Verification items for this drawing (mm, ordinates from the low corner). A direction names the side the tool comes from. Coordinates: 2 decimals unless noted, no trailing zeros.
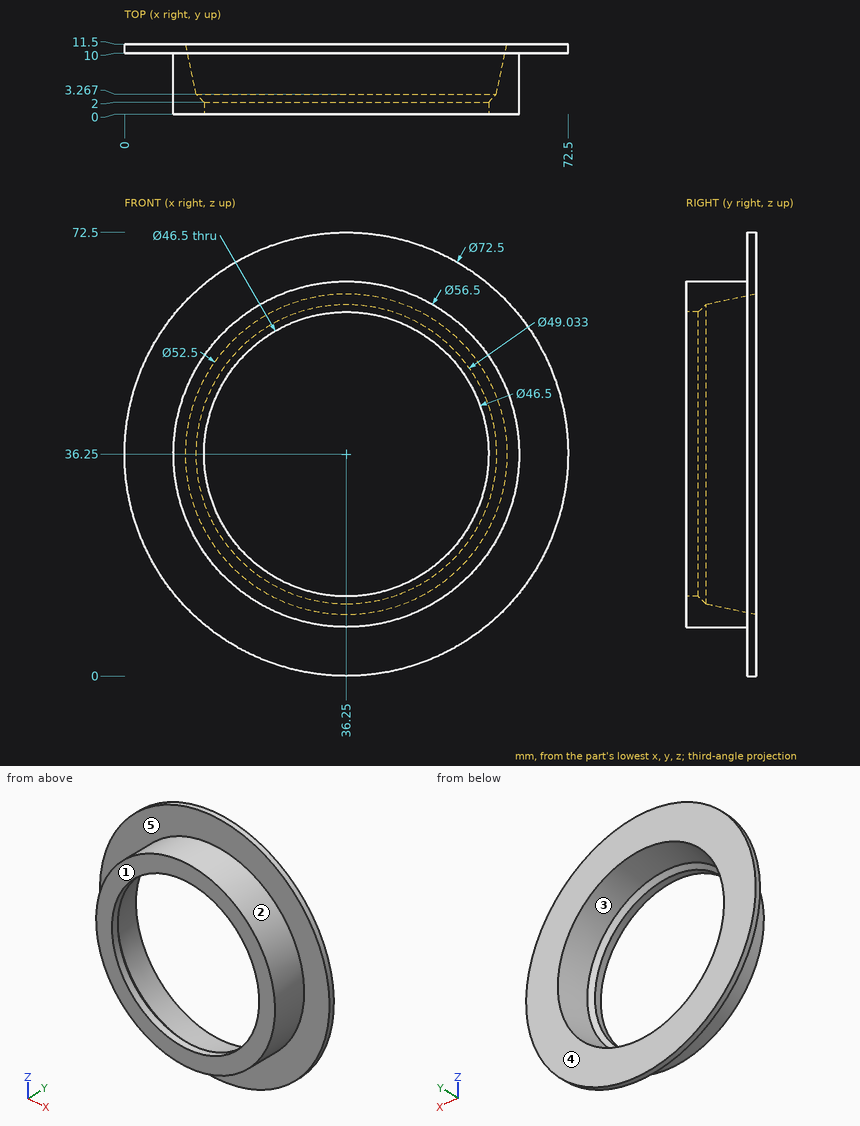
(1) Go/stop test with flat-tipped pins: P1, Ø12, axis at x = 32.5, z = 23, coming from the -Y side; P2, Ø1, axis at x = 15, y = 4, coming from the +Z side. Record where each tip stops, or that it passes through.
Filled in:
P1: passes through
P2: stops at z = 55.42
(2) Release check for a two-part mould opening along X. For the marked faces 1, 2 and 3 record: +X half, -X half, draft (parallel to the pull), parting line (faces both ways), or undercut.
Filled in:
face 1: draft
face 2: parting line
face 3: undercut
(3) Thickness scan on probe 1 along X at (y, z) = (1.1, 36.25); probe 2 along Z at (x, y) = (58, 4.25) (1 decimal). Record the ranges inside material, lowest first.
Filled in:
probe 1: x = 8 to 13, 59.5 to 64.5
probe 2: z = 18.2 to 24.5, 48 to 54.3
(4) Tool access check on the marked faces 4 and 5. Record the directions out of +Z, -Z, +X, -X, +Y, -Y that give a thin tool (end or side, any length) a straight path to the whole face; none if there is none.
Filled in:
face 4: +Z, -Z, +X, -X, +Y
face 5: -Y
